Could you check a few things on this model? Use its own coordinates, in mm. A direction names the side the tool comes from. Round coordinates to 2 decimals unless told otherwise and drop trailing zeros. Loops run counter-clockwise (first coordinate to the right, second up) from the corner with the lowest first, then second, coordinate; pieces in that order, holes last.
from build123d import *

# Parameters (mm, degrees)
SKETCH1_W                             = 35
SKETCH1_H                             = 26
BOSS_EXTRUDE1_DEPTH                   = 8
M3_CLEARANCE_HOLE1_D                  = 3.4
M3_CLEARANCE_HOLE1_DEPTH              = 8
M3_CLEARANCE_HOLE1_CSINK_D            = 3.45
M3_CLEARANCE_HOLE1_CSINK_ANGLE        = 90
M3_CLEARANCE_HOLE1_TIP                = 1.021463052
SKETCH6_R                             = 10.2
CUT_EXTRUDE1_DEPTH                    = 3.1
SKETCH7_R                             = 9
CUT_EXTRUDE2_DEPTH                    = 44.874935897
SKETCH8_R                             = 2.5
CUT_EXTRUDE3_DEPTH                    = 3.1
TAP_DRILL_FOR_M3X0_5_TAP1_D           = 2.5
TAP_DRILL_FOR_M3X0_5_TAP1_CSINK_D     = 2.55
TAP_DRILL_FOR_M3X0_5_TAP1_CSINK_ANGLE = 90
SKETCH11_W                            = 2.6
SKETCH11_H                            = 5.8
CUT_EXTRUDE4_DEPTH                    = 45.328320519


with BuildPart() as part:
    # Sketch1 → Boss-Extrude1 (new body)
    with BuildSketch(Plane(origin=(0, 0, 0), x_dir=(1, 0, 0), z_dir=(0, 1, 0))):
        with Locations((17.5, 13)):
            Rectangle(SKETCH1_W, SKETCH1_H)
    extrude(amount=BOSS_EXTRUDE1_DEPTH)

    # M3 Clearance Hole1
    with Locations(Plane(origin=(35, 0, 0), x_dir=(0, 0, -1), z_dir=(1, 0, 0))):
        with Locations((6, 5), (20, 5)):
            CounterSinkHole(M3_CLEARANCE_HOLE1_D / 2, M3_CLEARANCE_HOLE1_CSINK_D / 2, depth=M3_CLEARANCE_HOLE1_DEPTH, counter_sink_angle=M3_CLEARANCE_HOLE1_CSINK_ANGLE)
            with Locations((0, 0, -(M3_CLEARANCE_HOLE1_DEPTH + M3_CLEARANCE_HOLE1_TIP / 2))):  # 118° drill point
                Cone(0, M3_CLEARANCE_HOLE1_D / 2, M3_CLEARANCE_HOLE1_TIP, mode=Mode.SUBTRACT)

    # Sketch5 → Tap Drill for M22x1.5 Tap1 (revolve, cut)
    with BuildSketch(Plane(origin=(15, 0, -13), x_dir=(0, 0, -1), z_dir=(1, 0, 0))):
        Polygon((0, 0), (0, 3), (10.25, 3), (10.25, 0.025), (10.275, 0), align=None)
    revolve(axis=Axis((15, -6.35, -13), (0, 1, 0)), mode=Mode.SUBTRACT)

    # Sketch6 → Cut-Extrude1 (cut)
    with BuildSketch(Plane(origin=(0, 8, 0), x_dir=(1, 0, 0), z_dir=(0, 1, 0))):
        with Locations(Location((15, 13, 0), (0, 0, 270))):
            Circle(SKETCH6_R)
    extrude(amount=-CUT_EXTRUDE1_DEPTH, mode=Mode.SUBTRACT)

    # Sketch7 → Cut-Extrude2 (cut, through all)
    with BuildSketch(Plane(origin=(0, 4.9, 0), x_dir=(1, 0, 0), z_dir=(0, 1, 0))):
        with Locations(Location((15, 13, 0), (0, 0, 270))):
            Circle(SKETCH7_R)
    extrude(amount=-CUT_EXTRUDE2_DEPTH, mode=Mode.SUBTRACT)

    # Sketch8 → Cut-Extrude3 (cut)
    with BuildSketch(Plane(origin=(0, 8, 0), x_dir=(1, 0, 0), z_dir=(0, 1, 0))):
        with Locations((6, 17.8)):
            Circle(SKETCH8_R)
    extrude(amount=-CUT_EXTRUDE3_DEPTH, mode=Mode.SUBTRACT)

    # Tap Drill for M3x0.5 Tap1 (through all)
    with Locations(Plane(origin=(0, 8, 0), x_dir=(1, 0, 0), z_dir=(0, 1, 0))):
        with Locations((2.5, 23.5), (24.5, 23.5), (24.5, 2.5), (2.5, 2.5)):
            CounterSinkHole(TAP_DRILL_FOR_M3X0_5_TAP1_D / 2, TAP_DRILL_FOR_M3X0_5_TAP1_CSINK_D / 2, counter_sink_angle=TAP_DRILL_FOR_M3X0_5_TAP1_CSINK_ANGLE)

    # Sketch11 → Cut-Extrude4 (cut, through all)
    with BuildSketch(Plane(origin=(0, 8, 0), x_dir=(1, 0, 0), z_dir=(0, 1, 0))):
        with Locations((31.7, 6)):
            Rectangle(SKETCH11_W, SKETCH11_H)
        with Locations((31.7, 20)):
            Rectangle(SKETCH11_W, SKETCH11_H)
    extrude(amount=-CUT_EXTRUDE4_DEPTH, mode=Mode.SUBTRACT)


solid = part.part
Item 1: If we section it at B-B, the plane y = 1.25: Please give me the cut outline in (x, z).
Results list:
outline: (0, -26) - (35, -26) - (35, 0) - (0, 0) - close; hole circle Ø2.5 at (2.5, -23.5); hole circle Ø2.5 at (2.5, -2.5); hole circle Ø20.5 at (15, -13); hole circle Ø2.5 at (24.5, -23.5); hole circle Ø2.5 at (24.5, -2.5); hole (30.4, -22.9) - (33, -22.9) - (33, -17.1) - (30.4, -17.1) - close; hole (30.4, -8.9) - (33, -8.9) - (33, -3.1) - (30.4, -3.1) - close
Item 2: If we section it at D-D, the plane z = -17.75: Count the separate pieces of the cut face and the enclosed holes in it, then the cut area to 3 significant figures.
Results list:
separate pieces: 3
enclosed holes: 0
area: 112 mm2
Item 3: We'd pull the mould along X, two halves only. Please class faces 1 (the conical face through (26.156, 5.249, -6.159)), 2 (the flat face through (17, 4, -26)), 3 (the flat face through (11.2, 4.9, -21.4)): released by +X, released by -X, zero draft, split by the parting line, or undercut.
Results list:
face 1: released by +X
face 2: zero draft
face 3: undercut
Item 4: If I drill on line 1 along X through (y, z) = (6.45, -17.8); line 2 along X through (y, z) = (1.75, -2.25); line 3 along Z through (x, y) = (15, 3.5), over which ranges is the centre line in solid material (lowest first)?
Results list:
line 1: x = 0 to 3.5, 24 to 30.4, 33 to 35
line 2: x = 0 to 1.28, 3.72 to 23.28, 25.72 to 35
line 3: z = -26 to -22, -4 to 0
Item 5: If we section it at C-C, the plane x = 2.5: Please give me the cut outline in (y, z) (3 decimals).
Results list:
outline: (0, -26) - (8, -26) - (8, -24.775) - (7.975, -24.75) - (0, -24.75) - close; (0, -22.25) - (7.975, -22.25) - (8, -22.225) - (8, -3.775) - (7.975, -3.75) - (0, -3.75) - close; (0, -1.25) - (7.975, -1.25) - (8, -1.225) - (8, 0) - (0, 0) - close
Item 6: For faces 4 (the cylindrical face through (28.68, 3.34, -6.37)), 5 (the cylindrical face through (23.8, 6.47, -7.84)), 6 (the flat face through (32, 4, -3.1)), 7 (the cylindrical face through (25.006, 1.492, -10.778)), which set-ups out of +Z, -Z, +X, -X, +Y, -Y let a thin tool reach every point of the face, with its end or its side?
Results list:
face 4: +X
face 5: +Y
face 6: +Y, -Y
face 7: -Y
Item 7: Will these pins go through, and if not, where does the flat tip stop? pin 1 (1 mm diameter, centred on y = 6, z = -19.5, fed in from +X); pin 2 (2 mm diameter, centred on x = 19, z = -8.5, fed in from +Y); pin 3 (2 mm diameter, centred on y = 5, z = -20, fed in from +X).
Results list:
pin 1: stops at x = 26.95
pin 2: passes through
pin 3: stops at x = 26.58
Item 8: If we section it at A-A, the plane x = 15: Please give me the cut outline in (y, z) (3 decimals).
Results list:
outline: (0, -26) - (8, -26) - (8, -23.2) - (4.9, -23.2) - (4.9, -22) - (3, -22) - (3, -23.25) - (0.025, -23.25) - (0, -23.275) - close; (0, -2.725) - (0.025, -2.75) - (3, -2.75) - (3, -4) - (4.9, -4) - (4.9, -2.8) - (8, -2.8) - (8, 0) - (0, 0) - close
